```python
from build123d import *

# Parameters (mm, degrees)
BOSS_EXTRUDE1_DEPTH = 16
CHAMFER1_SIZE       = 2
SCALE2_SCALE        = 0.95


with BuildPart() as part:
    # Sketch1 → Boss-Extrude1 (new body)
    with BuildSketch(Plane.XY):
        Polygon((0, 18.847328042), (-4.053541246, 14.423664021), (-4.053541246, 4.423664021), (0, 0), (4.053541246, 4.423664021), (4.053541246, 14.423664021), align=None)
    extrude(amount=BOSS_EXTRUDE1_DEPTH)

    # Chamfer1
    chamfer1_edges = [part.edges().sort_by_distance(p)[0] for p in [
        (2.026770623, 16.635496031, 16),
        (-2.026770623, 16.635496031, 16),
        (-4.053541246, 9.423664021, 16),
        (-2.026770623, 2.21183201, 16),
        (2.026770623, 2.21183201, 16),
        (-2.026770623, 2.21183201, 0),
        (-4.053541246, 9.423664021, 0),
        (-2.026770623, 16.635496031, 0),
        (2.026770623, 16.635496031, 0),
        (4.053541246, 9.423664021, 0),
        (2.026770623, 2.21183201, 0),
        (4.053541246, 9.423664021, 16),
    ]]
    chamfer(chamfer1_edges, length=CHAMFER1_SIZE)


with BuildPart() as part_1:
    # Scale2: scaled about (0, 0, 0)
    add(part.part.scale(SCALE2_SCALE))


solid = part_1.part
```
Input: part model. Units: mm. Frame: model coordinates. Give positions to 0.01 mm unless a question says otherwise; leave off trailing zeros. Order: outer loops, then holes, each group sorted by start corner. A loop starts at its lowest first (then second) coordinate and runs counter-clockwise, first axis right, second up. Notation, with made-up numbers: (-18.75, 73.25) - (32.25, 73.25) arc R31 ccw to (32.25, 112.25) - close; hole circle Ø5 at (-18.5, -22.5). An arc over 180 degrees is marked (long way). One line per item, written item: value.
1. Cut plane B-B, the plane y = 8.25. Output: boundary loops of the cut face in (x, z), and give its area (3 significant figures).
Determined:
outline: (-3.85, 1.9) - (-1.95, 0) - (1.95, 0) - (3.85, 1.9) - (3.85, 13.3) - (1.95, 15.2) - (-1.95, 15.2) - (-3.85, 13.3) - close
area: 110 mm2
2. Line query: probe 1 along Y at (x, z) = (-2.75, 2.25); probe 2 along Y at (x, z) = (2.5, 8.25); probe 3 along X at (y, z) = (16.75, 6). Output: solid intervals per line, ascending.
Determined:
probe 1: 3 to 14.9
probe 2: 2.73 to 15.18
probe 3: -1.06 to 1.06
3. Cut plane D-D, the plane z = 14.25. Output: boundary loops of the cut face in (x, y), and give its area (3 significant figures).
Determined:
outline: (-2.9, 4.57) - (0, 1.41) - (2.9, 4.57) - (2.9, 13.33) - (0, 16.5) - (-2.9, 13.33) - close
area: 69.2 mm2
4. Cut plane A-A, the plane x = 2.25. Output: boundary loops of the cut face in (y, z), and give its area (3 significant figures).
Determined:
outline: (2.46, 1.9) - (4.83, 0.3) - (13.08, 0.3) - (15.45, 1.9) - (15.45, 13.3) - (13.08, 14.9) - (4.83, 14.9) - (2.46, 13.3) - close
area: 182 mm2
5. Pin query (flat end, axial travel): pin 1 Ø2 at (x, y) = (1, 3) entering from +Z. Return the tip coordinate at first contact, or that it passes through.
Determined:
pin 1: z = 15.2
6. Cut plane C-C, the plane z = 11. Output: boundary loops of the cut face in (x, y).
Determined:
outline: (-3.85, 4.2) - (0, 0) - (3.85, 4.2) - (3.85, 13.7) - (0, 17.9) - (-3.85, 13.7) - close
